For this review, use the dimensioned drawing (mm, ordinates from the lowest corner) and the shaded views. A direction names the side the tool comes from. Round coordinates to 2 decimals unless told otherwise and drop trailing zeros. Write each loop counter-clockwise with the first axis right and the second up, starting at its lowest first coordinate (ties: lowest second). Pieces come first, ordered by that corner, then holes. Notation, with made-up numbers: M -11.5,54 L 20.5,54 A21 ccw 20.5,58 Z; hole C 45.25,-11.75 d2. An arc over 180 degrees is marked long. Use one line per item in the form item = value. Start each with the question number.
Item 1: Draft analysis for pull direction Y (two halves, no side actions). For the marked faces 1, 2 and 3, state which applies: released by +Y, released by -Y, zero draft, split by the parting line, or undercut.
Item 2: Add section B-B (x = 7.5). State the section outline as (y, z) points, and give its area (3 significant figures).
Item 3: For line 1 (Y direction, x = 11.25, z = 2.5); line 2 (X direction, y = 119, z = 9.75); line 3 (Z direction, x = 8, y = 56.5), list the stretches that pass through material, from the lowest coordinate up. Write a range as [from, to].
Item 4: Add section A-A (z = 7.5). State the section outline as (x, y) points.
Item 5: Add section C-C (y = 36.5). State the section outline as (x, z) points, and give its area (3 significant figures).
Item 6: For P1, Ø1.5, axis at y = 66.5, z = 12, coming from the -X side; P2, Ø5, axis at y = 64, z = 8.5, coming from the -X side, all flat-tipped, find the tip position at first contact; note any pin that passes through.
Item 7: For the marked faces 4 and 5, list the 3-axis set-ups (+Z, -Z, +X, -X, +Y, -Y) from which the entire face can be reached by the end or side of a thin tool; tool diameter is ignored.
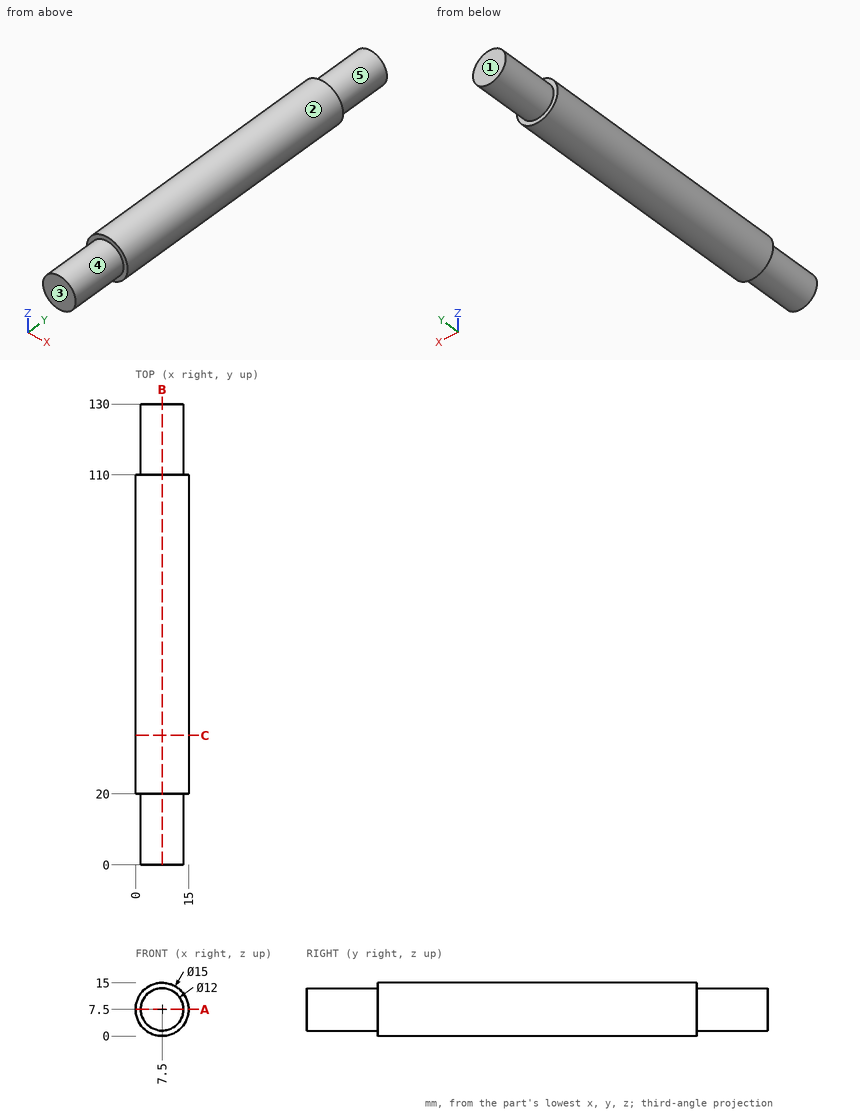
Calculated:
q1.face_1 = released by +Y
q1.face_2 = zero draft
q1.face_3 = released by -Y
q2.outline = M 0,1.5 L 20,1.5 L 20,0 L 110,0 L 110,1.5 L 130,1.5 L 130,13.5 L 110,13.5 L 110,15 L 20,15 L 20,13.5 L 0,13.5 Z
q2.area = 1,830 mm^2
q3.line_1 = [20, 110]
q3.line_2 = [1.94, 13.06]
q3.line_3 = [0.02, 14.98]
q4.outline = M 0,20 L 1.5,20 L 1.5,0 L 13.5,0 L 13.5,20 L 15,20 L 15,110 L 13.5,110 L 13.5,130 L 1.5,130 L 1.5,110 L 0,110 Z
q5.outline = C 7.5,7.5 d15
q5.area = 177 mm^2
q6.P1 = 1
q6.P2 = 0
q7.face_4 = -Y
q7.face_5 = +Y
